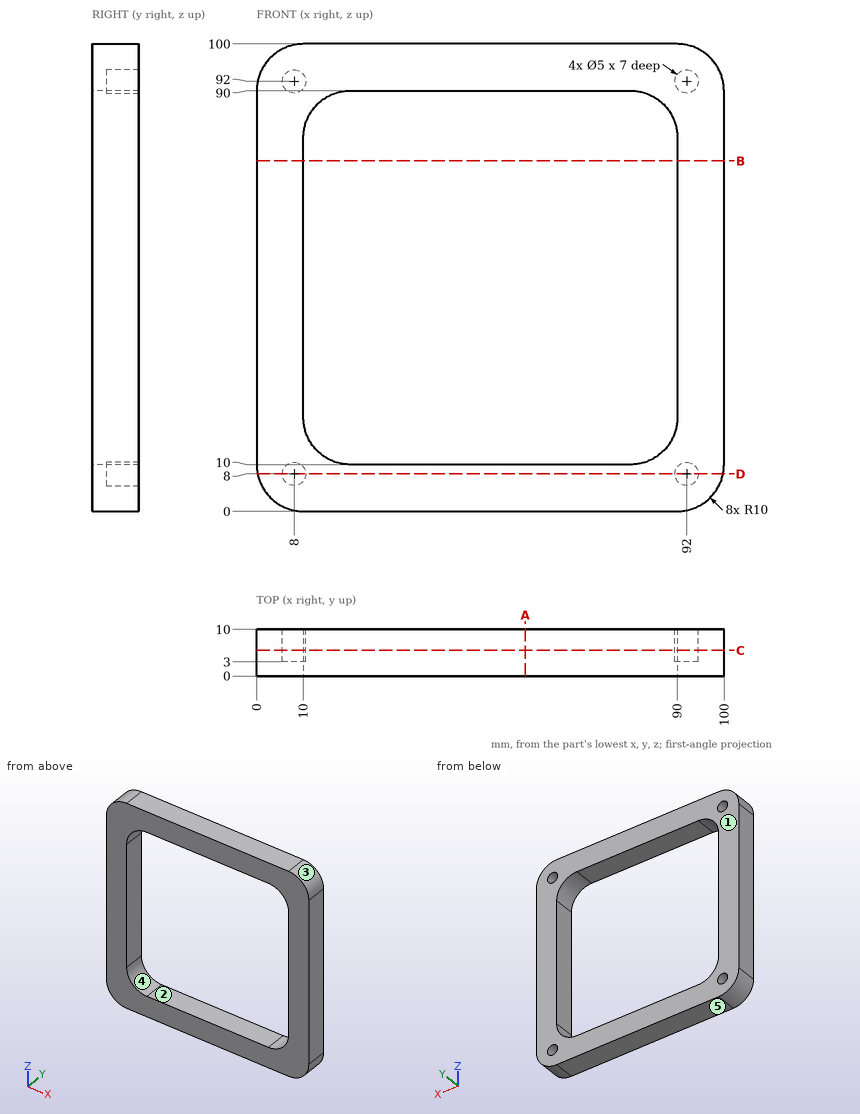
Design review of the part shown in the three views and the two pictorial views. Dimensions are in mm from the part's minimum x, y and z. A direction names the side the tool comes from. Give positions to 0.01 mm unless a question says otherwise; leave off trailing zeros. Loops run counter-clockwise (first coordinate to the right, second up) from the corner with the lowest first, then second, coordinate; pieces in that order, holes last. Notation, with made-up numbers: M -20.75,73.25 L 16.25,73.25 A27 ccw 16.25,92.25 Z; hole C 34,10 d8. An arc over 180 degrees is marked long. Answer as a JSON object with one key per item and string values. Group by question number.
Q1. Add section B-B on z = 75. Give the boundary of the cut face in (x, y).
Q2. Add section C-C on y = 5.5. Give the boundary of the cut face in (x, z), and give its area (3 significant figures).
Q3. Tool access review of the marked faces 1 and 2: name each direction out of +Z, -Z, +X, -X, +Y, -Y from which nothing blocks a thin tool from reaching the whole face with its end or side.
Q4. Mouldability with a two-part tool opening along X and no side actions: class the marked faces 3, 4 and 5 as +X half, -X half, draft (parallel to the pull), parting line (faces both ways), or undercut.
Q5. Insertion check: P1, Ø8, axis at x = 27, z = 16, coming from the +Y side; P2, Ø2.5, axis at x = 8, z = 7, coming from the +Y side. Each pin has a flat end and moves straight along its axis. Give the tip position at first contact, or say it passes through.
Q6. Add section D-D on z = 8. Give the boundary of the cut face in (x, y).
Q7. Add section A-A on x = 57.5. Give the boundary of the cut face in (y, z).
Q8. For probe 1 along X at (y, z) = (1.75, 20.5); probe 2 along X at (y, z) = (7, 92), list the stretches that pass through material, from the lowest coordinate up. Write a range as [from, to].
Checked values:
{
 "1": {"outline": "M 0,0 L 10,0 L 10,10 L 0,10 Z; M 90,0 L 100,0 L 100,10 L 90,10 Z"},
 "2": {"outline": "M 0,10 A10 ccw 10,0 L 90,0 A10 ccw 100,10 L 100,90 A10 ccw 90,100 L 10,100 A10 ccw 0,90 Z; hole C 8,8 d5; hole C 8,92 d5; hole M 10,20 A10 ccw 20,10 L 80,10 A10 ccw 90,20 L 90,80 A10 ccw 80,90 L 20,90 A10 ccw 10,80 Z; hole C 92,8 d5; hole C 92,92 d5", "area": "3,520 mm²"},
 "3": {"face 1": "+Z, -Z, +X, -X, +Y", "face 2": "+Y, -Y"},
 "4": {"face 3": "+X half", "face 4": "undercut", "face 5": "draft"},
 "5": {"P1": "through", "P2": "y = 3"},
 "6": {"outline": "M 0.2,0 L 99.8,0 L 99.8,10 L 94.5,10 L 94.5,3 L 89.5,3 L 89.5,10 L 10.5,10 L 10.5,3 L 5.5,3 L 5.5,10 L 0.2,10 Z"},
 "7": {"outline": "M 0,0 L 10,0 L 10,10 L 0,10 Z; M 0,90 L 10,90 L 10,100 L 0,100 Z"},
 "8": {"probe 1": "[0, 10], [90, 100]", "probe 2": "[0.2, 5.5], [10.5, 89.5], [94.5, 99.8]"}
}
